Source: CAD feature listing. Evaluate the final solid. Frame: model axes, mm. A direction names the side the tool comes from. Round coordinates to 2 decimals unless told otherwise and drop trailing zeros. Order: outer loops, then holes, each group sorted by start corner. A loop starts at its lowest first (then second) coordinate and runs counter-clockwise, first axis right, second up. Notation, with made-up numbers: (5, 83) - (19, 83) arc R32 ccw to (19, 120) - close; hole circle Ø2 at (-14, -23.75). An arc over 180 degrees is marked (long way). Return JSON: item names as keys, results as strings. Group by question number.
1) Mould query, pull axis Y, two halves, no side actions, for faces 1 (the flat face through (-57, -46, 0)), 2 (the flat face through (-57, -87.55, 25)), 3 (the flat face through (-57, -5.55, 25)), 4 (the flat face through (16.102, -47, 25)). Classes: pulls with the +Y half, pulls with the -Y half, needs draft (parallel to the pull), parting line crosses it, or undercut.
2) Access query for faces 5 (the flat face through (-128.898, -47, 25)), 6 (the flat face through (17.102, -47, 25)). Directions: +Z, -Z, +X, -X, +Y, -Y. A direction counts if a zero-diameter tool reaches every point of the face in a straight line with its end or side. Return the directions, or none.
3) Section C-C, the plane y = -12. Return loops of the section in (x, z).
4) Contact query for a flat-ended pin moving along its axis: P1, Ø12, axis at x = -76.5, y = -24, coming from the +Z side. Output: stop coordinate, or through.
5) Section A-A, the plane z = 26.5. Return loops of the section in (x, y).
6) Section B-B, the plane x = -97. Return loops of the section in (y, z).
7) Ray query, line 1 (X direction, y = -65, z = 18.5); line 2 (Y direction, x = -77.5, z = 27.5); line 3 (Z direction, x = -39, y = -13). Return the intervals inside material, ascending. Write a range as from..to.
```python
from build123d import *

# Parameters (mm, degrees)
F0_W     = 147
F0_H     = 82
F1_DEPTH = 50
F2_T     = -1


with BuildPart() as f1:
    # F0 (on Top) → F1 (new body)
    with BuildSketch(Plane.XY):
        with Locations((-95.298209, -46.550309)):
            Rectangle(F0_W, F0_H)
    extrude(amount=F1_DEPTH)

    # F2
    f2_openings = [f1.faces().sort_by_distance(p)[0] for p in [
        (-95.298209, -46.550309, 50),
    ]]
    offset(amount=F2_T, openings=f2_openings)


with BuildPart() as f1_1:
    # F3: moved
    add(f1.part.moved(Location((38.9, 0, 0))))


solid = f1_1.part
```
Geometry check:
{
 "1": {"face 1": "needs draft", "face 2": "pulls with the -Y half", "face 3": "pulls with the +Y half", "face 4": "undercut"},
 "2": {"face 5": "+Z", "face 6": "+Z, -Z, +X, +Y, -Y"},
 "3": {"outline": "(-129.9, 0) - (17.1, 0) - (17.1, 50) - (16.1, 50) - (16.1, 1) - (-128.9, 1) - (-128.9, 50) - (-129.9, 50) - close"},
 "4": {"P1": "z = 1"},
 "5": {"outline": "(-129.9, -87.55) - (17.1, -87.55) - (17.1, -5.55) - (-129.9, -5.55) - close; hole (-128.9, -86.55) - (16.1, -86.55) - (16.1, -6.55) - (-128.9, -6.55) - close"},
 "6": {"outline": "(-87.55, 0) - (-5.55, 0) - (-5.55, 50) - (-6.55, 50) - (-6.55, 1) - (-86.55, 1) - (-86.55, 50) - (-87.55, 50) - close"},
 "7": {"line 1": "-129.9..-128.9, 16.1..17.1", "line 2": "-87.55..-86.55, -6.55..-5.55", "line 3": "0..1"}
}
